Can you work these out from the model? Positions are in its coordinate system, mm. Face numbers are marked on the shaded views. A direction names the side the tool comes from. Give positions to 0.01 mm unless a question says otherwise; leave off trailing zeros. Order: outer loops, then holes, each group sorted by start corner. A loop starts at its lowest first (then second) coordinate and runs counter-clockwise, first axis right, second up. Notation, with made-up numbers: M 68.25,60.25 L 112.25,60.25 A21 cw 112.25,85.25 Z; hole C -37.75,16.25 d11. An arc over 180 degrees is marked long. Use one line per item in the form item = value. Start each with the question number.
1. We'd pull the mould along X, two halves only. Please class the marked faces 6, 7 and 8: +X half, -X half, draft (parallel to the pull), parting line (faces both ways), or undercut.
2. I need wall thicknesses on L1, parallel to X at y = 9.2, z = 0; L2, parallel to X at y = 5, z = -0.35; L3, parallel to X at y = 5.75, z = 0.65. Which ranges of each line are inside material? Lowest first, please.
3. For the marked faces 1, 2, 3, 4 and 5, which set-ups out of +Z, -Z, +X, -X, +Y, -Y let a thin tool reach every point of the face, with its end or its side?
4. Will these pins go through, and if not, where does the flat tip stop? P1, Ø2.5, axis at x = -2.5, z = 0, coming from the +Y side; P2, Ø1.9, axis at x = 1.5, y = 1.5, coming from the +Z side; P3, Ø1, axis at x = -2.5, z = 0, coming from the -Y side; P4, Ø0.6, axis at x = 2.5, z = -0.5, coming from the -Y side.
5. I want a section at C-C, the plane y = 2.75. List the corners of the cut face in (x, z) for me (3 decimals), and give its area (3 significant figures).
6. I want a section at A-A, the plane y = 6. List the corners of the cut face in (x, z) for me, and give its area (3 significant figures).
7. I want a section at B-B, the plane y = -1. List the corners of the cut face in (x, z) for me (3 decimals), and give its area (3 significant figures).
```python
from build123d import *

# Parameters (mm, degrees)
BOSS_EXTRUDE1_DEPTH = 9.4
SKETCH2_R           = 1
CUT_EXTRUDE1_DEPTH  = 6
SKETCH3_R           = 1.45
CUT_EXTRUDE2_DEPTH  = 0.5
CUT_EXTRUDE3_DEPTH  = 1
CUT_EXTRUDE4_REACH  = 10.277
FILLET1_START       = 1
FILLET1_DEPTH       = 2.4
FILLET1_START_2     = 3.146512
FILLET1_2_DEPTH     = 6.253488
SKETCH6_R           = 1.225
SKETCH6_R_2         = 0.625
BOSS_EXTRUDE2_DEPTH = 4
SKETCH7_W           = 1.225
SKETCH7_H           = 2.45
CUT_EXTRUDE5_DEPTH  = 2.3
CUT_EXTRUDE6_DEPTH  = 2.4


with BuildPart() as part:
    # Sketch1 → Boss-Extrude1 (new body)
    with BuildSketch(Plane(origin=(0, 0, 0), x_dir=(1, 0, 0), z_dir=(0, 1, 0))):
        Polygon((5.075, 1.6), (4.075, 2.6), (-5.075, 2.6), (-5.075, -2.6), (4.075, -2.6), (5.075, -1.6), align=None)
    extrude(amount=BOSS_EXTRUDE1_DEPTH)

    # Sketch2 → Cut-Extrude1 (cut)
    # profile 1 of 3: a face of its own
    with BuildSketch(Plane(origin=(0, 9.4, 0), x_dir=(1, 0, 0), z_dir=(0, 1, 0))):
        Polygon((4.075, -2.6), (5.075, -1.6), (5.075, 1.6), (4.075, 2.6), (-5.075, 2.6), (-5.075, -2.6), align=None)
        with BuildLine():
            Line((-2.5, -1.95), (-4.45, -1.95))
            Line((-4.45, -1.95), (-4.45, 1.95))
            Line((-4.45, 1.95), (-2.5, 1.95))
            ThreePointArc((-2.5, 1.95), (-1.270670915, 1.51368755), (-0.591466532, 0.4))
            Line((-0.591466532, 0.4), (0.591466532, 0.4))
            ThreePointArc((0.591466532, 0.4), (4.45, 0), (0.591466532, -0.4))
            Line((0.591466532, -0.4), (-0.591466532, -0.4))
            ThreePointArc((-0.591466532, -0.4), (-1.270670915, -1.51368755), (-2.5, -1.95))
        make_face(mode=Mode.SUBTRACT)
    # profile 2 of 3: a face of its own
    with BuildSketch(Plane(origin=(0, 9.4, 0), x_dir=(1, 0, 0), z_dir=(0, 1, 0))):
        with Locations(Location((2.5, 0, 0), (0, 0, 270))):
            Circle(SKETCH2_R)
    # profile 3 of 3: a face of its own
    with BuildSketch(Plane(origin=(0, 9.4, 0), x_dir=(1, 0, 0), z_dir=(0, 1, 0))):
        with Locations(Location((-2.5, 0, 0), (0, 0, 270))):
            Circle(SKETCH2_R)
    extrude(amount=-CUT_EXTRUDE1_DEPTH, mode=Mode.SUBTRACT)

    # Sketch3 → Cut-Extrude2 (cut)
    with BuildSketch(Plane(origin=(0, 9.4, 0), x_dir=(1, 0, 0), z_dir=(0, 1, 0))):
        with Locations(Location((-2.5, 0, 0), (0, 0, 270))):
            Circle(SKETCH3_R)
        with Locations(Location((2.5, 0, 0), (0, 0, 270))):
            Circle(SKETCH3_R)
    extrude(amount=-CUT_EXTRUDE2_DEPTH, mode=Mode.SUBTRACT)

    # Sketch4 → Cut-Extrude3 (cut)
    with BuildSketch(Plane.XZ):
        Polygon((3.826471863, 2), (-4.475, 2), (-4.475, -2), (3.826471863, -2), (4.475, -1.351471863), (4.475, 1.351471863), align=None)
    extrude(amount=-CUT_EXTRUDE3_DEPTH, mode=Mode.SUBTRACT)

    # Sketch5 → Cut-Extrude4 (cut, up to next)
    with BuildSketch(Plane(origin=(0, 3.4, 0), x_dir=(1, 0, 0), z_dir=(0, 1, 0)), mode=Mode.PRIVATE) as cut_extrude4_sk1:
        with BuildLine():
            Line((2.5, 1.95), (-2.5, 1.95))
            ThreePointArc((-2.5, 1.95), (-1.270670915, 1.51368755), (-0.591466532, 0.4))
            Line((-0.591466532, 0.4), (0.591466532, 0.4))
            ThreePointArc((0.591466532, 0.4), (1.270670915, 1.51368755), (2.5, 1.95))
        make_face()
    cut_extrude4_tool1 = extrude(cut_extrude4_sk1.sketch, amount=-CUT_EXTRUDE4_REACH, mode=Mode.PRIVATE) & part.part
    # Sketch5 → Cut-Extrude4 (cut, up to next)
    with BuildSketch(Plane(origin=(0, 3.4, 0), x_dir=(1, 0, 0), z_dir=(0, 1, 0)), mode=Mode.PRIVATE) as cut_extrude4_sk2:
        with BuildLine():
            Line((-2.5, -1.95), (2.5, -1.95))
            ThreePointArc((2.5, -1.95), (1.270670915, -1.51368755), (0.591466532, -0.4))
            Line((0.591466532, -0.4), (-0.591466532, -0.4))
            ThreePointArc((-0.591466532, -0.4), (-1.270670915, -1.51368755), (-2.5, -1.95))
        make_face()
    cut_extrude4_tool2 = extrude(cut_extrude4_sk2.sketch, amount=-CUT_EXTRUDE4_REACH, mode=Mode.PRIVATE) & part.part
    add(cut_extrude4_tool1.solids().sort_by_distance((0, 3.4, -1.344451))[0], mode=Mode.SUBTRACT)
    add(cut_extrude4_tool2.solids().sort_by_distance((0, 3.4, 1.344451))[0], mode=Mode.SUBTRACT)

    # Fillet1: read off the stored shape, not the designer's step
    # Fillet1 outline → Fillet1 (add)
    with BuildSketch(Plane(origin=(0, 0, 0), x_dir=(1, 0, 0), z_dir=(0, 1, 0)).offset(FILLET1_START)):
        with BuildLine():
            ThreePointArc((1.36718641, 1.587209302), (1.905255576, 1.85708887), (2.5, 1.95))
            Line((2.5, 1.95), (1.2510004, 1.95))
            ThreePointArc((1.2510004, 1.95), (1.441471054, 1.810999428), (1.36718641, 1.587209302))
        make_face()
        with BuildLine():
            ThreePointArc((1.36718641, -1.587209302), (1.441471054, -1.810999428), (1.2510004, -1.95))
            Line((1.2510004, -1.95), (2.5, -1.95))
            ThreePointArc((2.5, -1.95), (1.905255576, -1.85708887), (1.36718641, -1.587209302))
        make_face()
        with BuildLine():
            Line((-2.5, -1.95), (-1.2510004, -1.95))
            ThreePointArc((-1.2510004, -1.95), (-1.441471054, -1.810999428), (-1.36718641, -1.587209302))
            ThreePointArc((-1.36718641, -1.587209302), (-1.905255576, -1.857088869), (-2.5, -1.95))
        make_face()
        with BuildLine():
            ThreePointArc((0.435417718, -0.4), (0.555495212, -0.44005815), (0.627471884, -0.544186047))
            ThreePointArc((0.627471884, -0.544186047), (0.608095119, -0.472436154), (0.591466532, -0.4))
            Line((0.591466532, -0.4), (0.435417718, -0.4))
        make_face()
        with BuildLine():
            ThreePointArc((-0.591466532, -0.4), (-0.608095119, -0.472436154), (-0.627471884, -0.544186047))
            ThreePointArc((-0.627471884, -0.544186047), (-0.555495212, -0.44005815), (-0.435417718, -0.4))
            Line((-0.435417718, -0.4), (-0.591466532, -0.4))
        make_face()
        with BuildLine():
            ThreePointArc((-1.36718641, 1.587209302), (-1.441471054, 1.810999428), (-1.2510004, 1.95))
            Line((-1.2510004, 1.95), (-2.5, 1.95))
            ThreePointArc((-2.5, 1.95), (-1.905255576, 1.857088869), (-1.36718641, 1.587209302))
        make_face()
        with BuildLine():
            ThreePointArc((0.591466532, 0.4), (0.608095119, 0.472436154), (0.627471884, 0.544186047))
            ThreePointArc((0.627471884, 0.544186047), (0.555495212, 0.44005815), (0.435417718, 0.4))
            Line((0.435417718, 0.4), (0.591466532, 0.4))
        make_face()
        with BuildLine():
            ThreePointArc((-0.435417718, 0.4), (-0.555495212, 0.44005815), (-0.627471884, 0.544186047))
            ThreePointArc((-0.627471884, 0.544186047), (-0.608095119, 0.472436154), (-0.591466532, 0.4))
            Line((-0.591466532, 0.4), (-0.435417718, 0.4))
        make_face()
    extrude(amount=FILLET1_DEPTH)

    # Fillet1 2 outline → Fillet1 2 (add)
    with BuildSketch(Plane(origin=(0, 0, 0), x_dir=(1, 0, 0), z_dir=(0, 1, 0)).offset(FILLET1_START_2)):
        with BuildLine():
            ThreePointArc((0.435417718, -0.4), (0.555495212, -0.44005815), (0.627471884, -0.544186047))
            ThreePointArc((0.627471884, -0.544186047), (0.608095119, -0.472436154), (0.591466532, -0.4))
            Line((0.591466532, -0.4), (0.435417718, -0.4))
        make_face()
        with BuildLine():
            ThreePointArc((-0.591466532, -0.4), (-0.608095119, -0.472436154), (-0.627471884, -0.544186047))
            ThreePointArc((-0.627471884, -0.544186047), (-0.555495212, -0.44005815), (-0.435417718, -0.4))
            Line((-0.435417718, -0.4), (-0.591466532, -0.4))
        make_face()
        with BuildLine():
            ThreePointArc((0.591466532, 0.4), (0.608095119, 0.472436154), (0.627471884, 0.544186047))
            ThreePointArc((0.627471884, 0.544186047), (0.555495212, 0.44005815), (0.435417718, 0.4))
            Line((0.435417718, 0.4), (0.591466532, 0.4))
        make_face()
        with BuildLine():
            ThreePointArc((-0.435417718, 0.4), (-0.555495212, 0.44005815), (-0.627471884, 0.544186047))
            ThreePointArc((-0.627471884, 0.544186047), (-0.608095119, 0.472436154), (-0.591466532, 0.4))
            Line((-0.591466532, 0.4), (-0.435417718, 0.4))
        make_face()
    extrude(amount=FILLET1_2_DEPTH)

    # Sketch6 → Boss-Extrude2 (add)
    # profile 1 of 2: a face of its own
    with BuildSketch(Plane.XZ.offset(-1)):
        with Locations(Location((-2.5, 0, 0), (0, 0, 90))):
            Circle(SKETCH6_R)
        with Locations(Location((-2.5, 0, 0), (0, 0, 270))):
            Circle(SKETCH6_R_2, mode=Mode.SUBTRACT)
    # profile 2 of 2: a face of its own
    with BuildSketch(Plane.XZ.offset(-1)):
        with Locations(Location((2.5, 0, 0), (0, 0, 90))):
            Circle(SKETCH6_R)
        with Locations(Location((2.5, 0, 0), (0, 0, 90))):
            Circle(SKETCH6_R_2, mode=Mode.SUBTRACT)
    extrude(amount=BOSS_EXTRUDE2_DEPTH)

    # Sketch7 → Cut-Extrude5 (cut)
    with BuildSketch(Plane.XZ.offset(3)):
        with Locations((-3.1125, 0)):
            Rectangle(SKETCH7_W, SKETCH7_H)
        with Locations((3.1125, 0)):
            Rectangle(SKETCH7_W, SKETCH7_H)
    extrude(amount=-CUT_EXTRUDE5_DEPTH, mode=Mode.SUBTRACT)

    # Sketch8 → Cut-Extrude6 (cut)
    with BuildSketch(Plane(origin=(0, 0.5, 0), x_dir=(-1, 0, 0), z_dir=(0, -1, 0))):
        Polygon((-4.075, -2.6), (5.075, -2.6), (5.075, 2.6), (-4.075, 2.6), (-5.075, 1.6), (-5.075, -1.6), align=None)
        Polygon((-3.992157288, -2.4), (4.875, -2.4), (4.875, 2.4), (-3.992157288, 2.4), (-4.875, 1.517157288), (-4.875, -1.517157288), align=None, mode=Mode.SUBTRACT)
    extrude(amount=-CUT_EXTRUDE6_DEPTH, mode=Mode.SUBTRACT)


solid = part.part
```
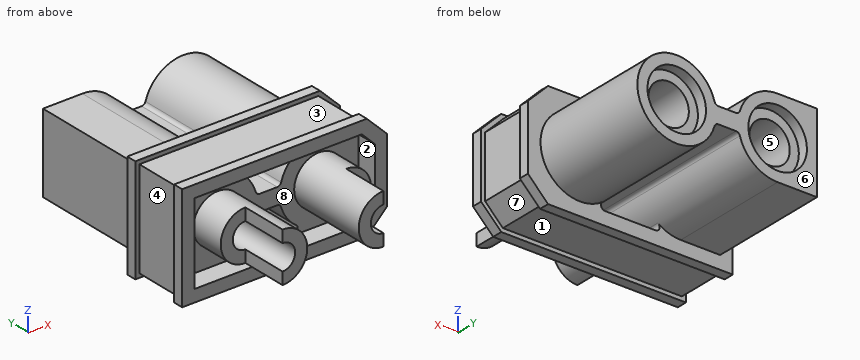
Check result:
q1.face_6 = draft
q1.face_7 = +X half
q1.face_8 = undercut
q2.L1 = -4.45 to -3.95, -1.05 to 1.05, 3.95 to 4.45
q2.L2 = -4.45 to -3.44, -1.56 to 1.56, 3.44 to 4.42
q2.L3 = -4.45 to -3.26, -1.74 to -0.66, 0.66 to 1.74, 3.26 to 4.34
q3.face_1 = -Z, +X, -X
q3.face_2 = -Y
q3.face_3 = +Z, +X, -X
q3.face_4 = +Z, -Z, -X
q3.face_5 = +Y
q4.P1 = 8.9
q4.P2 = 2.4
q4.P3 = 1
q4.P4 = -3
q5.outline = M -4.875,-2.4 L 3.992,-2.4 L 4.875,-1.517 L 4.875,1.517 L 3.992,2.4 L -4.875,2.4 Z; hole M -1.367,-1.587 A0.2 ccw -1.251,-1.95 L 1.251,-1.95 A0.2 ccw 1.367,-1.587 A1.95 cw 0.627,-0.544 A0.2 ccw 0.435,-0.4 L -0.435,-0.4 A0.2 ccw -0.627,-0.544 A1.95 cw Z; hole M -1.367,1.587 A1.95 cw -0.627,0.544 A0.2 ccw -0.435,0.4 L 0.435,0.4 A0.2 ccw 0.627,0.544 A1.95 cw 1.367,1.587 A0.2 ccw 1.251,1.95 L -1.251,1.95 A0.2 ccw Z
q5.area = 39.8 mm2
q6.outline = M -4.45,-1.95 L -2.5,-1.95 A1.95 ccw -0.63,-0.54 A0.2 cw -0.44,-0.4 L 0.44,-0.4 A0.2 cw 0.63,-0.54 A1.95 ccw long 0.63,0.54 A0.2 cw 0.44,0.4 L -0.44,0.4 A0.2 cw -0.63,0.54 A1.95 ccw -2.5,1.95 L -4.45,1.95 Z; hole C -2.5,0 d2; hole C 2.5,0 d2
q6.area = 20.2 mm2
q7.outline = M -2.5,-1.225 A1.225 ccw -2.5,1.225 L -2.5,0.625 A0.625 cw -2.5,-0.625 Z; M 2.5,-1.225 L 2.5,-0.625 A0.625 cw 2.5,0.625 L 2.5,1.225 A1.225 ccw Z
q7.area = 3.49 mm2
